Can you work these out from the model? Positions are in its coordinate system, mm. Face numbers are marked on the shaded views. A direction names the side the tool comes from. Coordinates: 2 decimals unless noted, no trailing zeros. Order: outer loops, then holes, each group sorted by start corner. A loop starts at its lowest first (then second) coordinate and runs counter-clockwise, first axis right, second up.
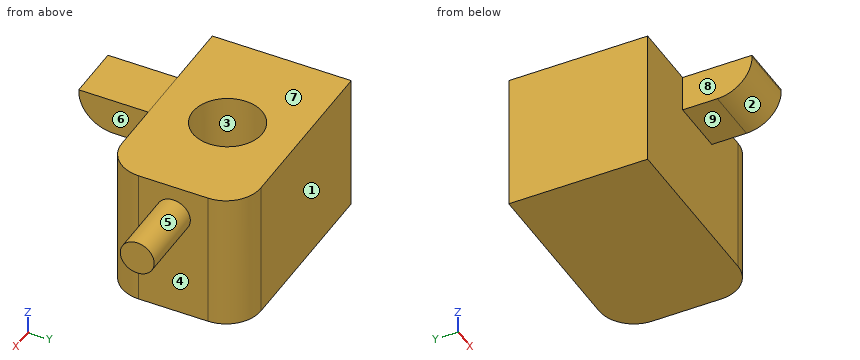
```python
from build123d import *

# Parameters (mm, degrees)
F0_W     = 76.2
F0_H     = 50.8
F1_DEPTH = 50.8
F2_R     = 12.7
F3_DEPTH = 25.4
F4_R     = 12.7
F5_W     = 20.487596
F5_H     = 13.337251
F6_DEPTH = 25.4
F7_R     = 12.7
F8_R     = 6.211161
F9_DEPTH = 25.4


with BuildPart() as f1:
    # F0 (on Top) → F1 (new body)
    with BuildSketch(Plane.XY):
        Rectangle(F0_W, F0_H)
    extrude(amount=F1_DEPTH)

    # F2 (on face) → F3 (cut)
    with BuildSketch(Plane.XY.offset(50.8)):
        Circle(F2_R)
    extrude(amount=-F3_DEPTH, mode=Mode.SUBTRACT)

    # F4
    f4_edges = [f1.edges().sort_by_distance(p)[0] for p in [
        (38.1, -25.4, 25.4),
        (38.1, 25.4, 25.4),
    ]]
    fillet(f4_edges, radius=F4_R)

    # F5 (on face) → F6 (join)
    with BuildSketch(Plane.XZ.offset(25.4)):
        with Locations((-3.261952, 44.131374)):
            Rectangle(F5_W, F5_H)
    extrude(amount=F6_DEPTH)

    # F7
    f7_edges = [f1.edges().sort_by_distance(p)[0] for p in [
        (-3.261952, -50.8, 37.462749),
    ]]
    fillet(f7_edges, radius=F7_R)

    # F8 (on face) → F9 (join)
    with BuildSketch(Plane.YZ.offset(38.1)):
        with Locations((0, 39.23849)):
            Circle(F8_R)
    extrude(amount=F9_DEPTH)


solid = f1.part
```
1. Imagine slicing it at A-A on z = 43. Please give me the cut outline in (x, y), then the cut area to 3 significant figures.
Completed:
outline: (-38.1, -25.4) - (-13.51, -25.4) - (-13.51, -48.59) - (6.98, -48.59) - (6.98, -25.4) - (25.4, -25.4) arc R12.7 ccw to (38.1, -12.7) - (38.1, -4.94) - (63.5, -4.94) - (63.5, 4.94) - (38.1, 4.94) - (38.1, 12.7) arc R12.7 ccw to (25.4, 25.4) - (-38.1, 25.4) - close; hole circle Ø25.4 at (0, 0)
area: 4,020 mm2
2. Please list where these lines run through material, in increasing order: probe 1 along Y at (x, z) = (0, 37.25); probe 2 along Y at (x, z) = (-3, 29.5); probe 3 along Z at (x, y) = (1, -37.5).
Completed:
probe 1: y = -25.4 to -12.7, 12.7 to 25.4
probe 2: y = -25.4 to -12.34, 12.34 to 25.4
probe 3: z = 37.46 to 50.8
3. Imagine slicing it at D-D on z = 16.5. Please give me the cut outline in (x, y).
Completed:
outline: (-38.1, -25.4) - (25.4, -25.4) arc R12.7 ccw to (38.1, -12.7) - (38.1, 12.7) arc R12.7 ccw to (25.4, 25.4) - (-38.1, 25.4) - close
4. Thinking about a two-plate mould opening in Y: for the marked faces 1, 2, 3 and 4, which applies, pulls with the +Y half, pulls with the -Y half, needs draft (parallel to the pull), parting line crosses it, or undercut?
Completed:
face 1: pulls with the +Y half
face 2: pulls with the -Y half
face 3: undercut
face 4: needs draft
5. Imagine slicing it at C-C on y = 0. Please give me the cut outline in (x, z), then the cut area to 3 significant figures.
Completed:
outline: (-38.1, 0) - (38.1, 0) - (38.1, 33.03) - (63.5, 33.03) - (63.5, 45.45) - (38.1, 45.45) - (38.1, 50.8) - (12.7, 50.8) - (12.7, 25.4) - (-12.7, 25.4) - (-12.7, 50.8) - (-38.1, 50.8) - close
area: 3,540 mm2
6. I'm going to push flat-ended pins straight in: pin 1 (5 mm diameter, centred on x = 35, z = 13.5, fed in from +Y); pin 2 (12.5 mm diameter, centred on x = -0.5, y = 6, fed in from +Z); pin 3 (1.5 mm diameter, centred on x = -10, z = 24, fed in from -Y). Where does each tip first touch, or does it pass through?
Completed:
pin 1: stops at y = 23.23
pin 2: stops at z = 25.4
pin 3: stops at y = -25.4
7. Imagine slicing it at B-B on x = 0. Please give me the cut outline in (y, z).
Completed:
outline: (-50.8, 50.16) arc R12.7 ccw to (-38.1, 37.46) - (-25.4, 37.46) - (-25.4, 0) - (25.4, 0) - (25.4, 50.8) - (12.7, 50.8) - (12.7, 25.4) - (-12.7, 25.4) - (-12.7, 50.8) - (-50.8, 50.8) - close
8. On a 3-axis mill with a long thin cutter (end or side, diameter ignored), from which of +Z, -Z, +X, -X, +Y, -Y can I reach the whole of each face in a straight line? I mean the marked faces 5, 6, 7, 8 and 9. Say none if no direction works.
Completed:
face 5: +X
face 6: +Z, -Z, +X, -Y
face 7: +Z, +X, -X, +Y, -Y
face 8: +Z, -Z, -X, -Y
face 9: -Z, +X, -X, -Y
